Design review of the part built by this model. Coordinates are the model's own, in mm. Coordinates: 2 decimals unless noted, no trailing zeros. Loops run counter-clockwise (first coordinate to the right, second up) from the corner with the lowest first, then second, coordinate; pieces in that order, holes last. Notation, with made-up numbers: (11, 37) - (17, 37) arc R10 ccw to (17, 50) - close; hole circle Ø2 at (11, -3.75). An arc over 180 degrees is marked (long way). One line per question, with ' | ' between items.
from build123d import *

# Parameters (mm, degrees)
SKETCH1_R           = 1.1
SKETCH1_R_2         = 3.7
SKETCH1_R_3         = 2
SKETCH1_W           = 5.85
SKETCH1_H           = 2.6
BOSS_EXTRUDE1_DEPTH = 3.175


with BuildPart() as part:
    # Sketch1 → Boss-Extrude1 (new body)
    with BuildSketch(Plane.XY):
        with BuildLine():
            Line((19, 0), (76, 0))
            Line((76, 0), (76, 32))
            Line((76, 32), (19, 32))
            ThreePointArc((19, 32), (3, 16), (19, 0))
        make_face()
        with Locations((8.25, 16)):
            Circle(SKETCH1_R, mode=Mode.SUBTRACT)
        with Locations((9.98438854, 25.01561146)):
            Circle(SKETCH1_R, mode=Mode.SUBTRACT)
        with Locations((28.01561146, 25.01561146)):
            Circle(SKETCH1_R, mode=Mode.SUBTRACT)
        with Locations((28.01561146, 6.98438854)):
            Circle(SKETCH1_R, mode=Mode.SUBTRACT)
        with Locations((9.98438854, 6.98438854)):
            Circle(SKETCH1_R, mode=Mode.SUBTRACT)
        with Locations((19, 26.75)):
            Circle(SKETCH1_R, mode=Mode.SUBTRACT)
        with Locations((29.75, 16)):
            Circle(SKETCH1_R, mode=Mode.SUBTRACT)
        with Locations((19, 5.25)):
            Circle(SKETCH1_R, mode=Mode.SUBTRACT)
        with Locations((19, 16)):
            Circle(SKETCH1_R_2, mode=Mode.SUBTRACT)
        with Locations((55, 5)):
            Circle(SKETCH1_R_3, mode=Mode.SUBTRACT)
        with Locations((55, 25.7)):
            Circle(SKETCH1_R_3, mode=Mode.SUBTRACT)
        with Locations((44.925, 25.7)):
            Rectangle(SKETCH1_W, SKETCH1_H, mode=Mode.SUBTRACT)
        with Locations((65.075, 25.7)):
            Rectangle(SKETCH1_W, SKETCH1_H, mode=Mode.SUBTRACT)
        with Locations((44.925, 5)):
            Rectangle(SKETCH1_W, SKETCH1_H, mode=Mode.SUBTRACT)
        with Locations((65.075, 5)):
            Rectangle(SKETCH1_W, SKETCH1_H, mode=Mode.SUBTRACT)
    extrude(amount=BOSS_EXTRUDE1_DEPTH)


solid = part.part
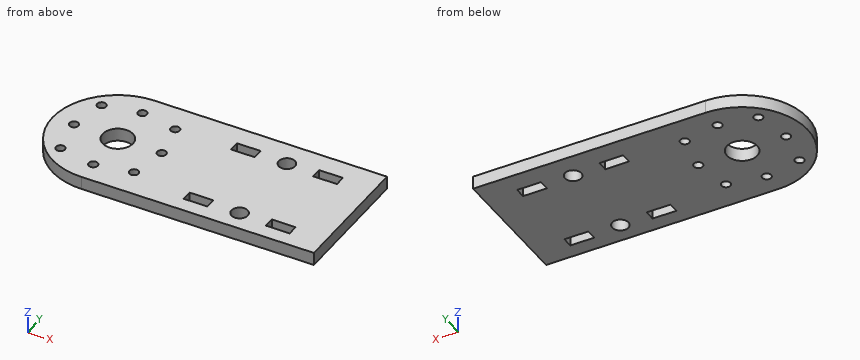
Q1. Take a section at B-B (z = 1.3). State how many separate pieces and enclosed holes the cut face has, plus the area to 3 significant figures.
Returned:
separate pieces: 1 | enclosed holes: 15 | area: 2,070 mm²
Q2. Take a section at C-C (y = 18). Give the boundary of the cut face in (x, z) (1 decimal), plus the area to 3 significant figures.
Returned:
outline: (3.1, 0) - (15.9, 0) - (15.9, 3.2) - (3.1, 3.2) - close; (22.1, 0) - (76, 0) - (76, 3.2) - (22.1, 3.2) - close | area: 212 mm²
Q3. To check wall thickness, follow line 1 along Y through (x, z) = (66.5, 0.45); line 2 along Y through (x, z) = (55, 1.55); line 3 along Y through (x, z) = (19, 1.55). State the ranges of each line that lie inside material, in increasing order.
Returned:
line 1: y = 0 to 3.7, 6.3 to 24.4, 27 to 32 | line 2: y = 0 to 3, 7 to 23.7, 27.7 to 32 | line 3: y = 0 to 4.15, 6.35 to 12.3, 19.7 to 25.65, 27.85 to 32
Q4. Take a section at D-D (y = 29). Give the boundary of the cut face in (x, z) (3 decimals), plus the area to 3 significant figures.
Returned:
outline: (9.673, 0) - (76, 0) - (76, 3.175) - (9.673, 3.175) - close | area: 211 mm²
Q5. Take a section at A-A (x = 55). Give the boundary of the cut face in (y, z) (3 decimals), plus the area to 3 significant figures.
Returned:
outline: (0, 0) - (3, 0) - (3, 3.175) - (0, 3.175) - close; (7, 0) - (23.7, 0) - (23.7, 3.175) - (7, 3.175) - close; (27.7, 0) - (32, 0) - (32, 3.175) - (27.7, 3.175) - close | area: 76.2 mm²
